```python
from build123d import *

# Parameters (mm, degrees)
F0_W      = 38.1
F0_H      = 38.1
F1_DEPTH  = 38.1
F6_DEPTH  = 38.1
F8_DEPTH  = 38.1
F9_W      = 25.4
F9_H      = 7.62
F10_DEPTH = 38.1


with BuildPart() as f1:
    # F0 (on Front) → F1 (new body)
    with BuildSketch(Plane.XZ):
        with Locations((19.05, 19.05)):
            Rectangle(F0_W, F0_H)
    extrude(amount=F1_DEPTH)

    # F5 (on offset) → F6 (cut)
    with BuildSketch(Plane.YZ.offset(38.1)):
        Polygon((-11.43, 15.875), (-6.35, 38.1), (-31.75, 38.1), (-26.67, 15.875), (-21.59, 28.575), (-16.51, 28.575), align=None)
        Polygon((-31.75, 0), (-38.1, 38.1), (-38.1, 0), align=None)
        Polygon((-25.4, 0), (-12.7, 0), (-19.05, 15.875), align=None)
        Polygon((-6.35, 0), (0, 0), (0, 38.1), align=None)
    extrude(amount=-F6_DEPTH, mode=Mode.SUBTRACT)

    # F7 (on Front) → F8 (cut)
    with BuildSketch(Plane.XZ):
        Polygon((11.43, 22.225), (6.35, 0), (31.75, 0), (26.67, 22.225), (21.59, 9.650744), (16.51, 9.525), align=None)
        Polygon((31.75, 38.1), (38.1, 0), (38.1, 38.1), align=None)
        Polygon((25.4, 38.1), (12.7, 38.1), (19.05, 22.225), align=None)
        Polygon((0, 38.1), (0, 0), (6.35, 38.1), align=None)
    extrude(amount=F8_DEPTH, mode=Mode.SUBTRACT)

    # F9 (on offset) → F10 (cut)
    with BuildSketch(Plane.XY.offset(38.1)):
        with Locations((25.4, -11.43)):
            Rectangle(F9_W, F9_H)
        with Locations((12.7, -26.67)):
            Rectangle(F9_W, F9_H)
    extrude(amount=-F10_DEPTH, mode=Mode.SUBTRACT)


solid = f1.part
```
Build history of the part. All positions in model axes, mm. A direction names the side the tool comes from. Coordinates: 2 decimals unless noted, no trailing zeros. Order: outer loops, then holes, each group sorted by start corner. A loop starts at its lowest first (then second) coordinate and runs counter-clockwise, first axis right, second up. Notation, with made-up numbers: (-25.75, -5.75) -> (21.25, -5.75) arc R24 ccw to (21.25, 6.25) -> close; hole circle Ø3 at (-11, -28). An arc over 180 degrees is marked (long way). Answer in a Markdown table with one row per item. Add a question column.
Q1. Band-saw the part on B-B, the plane z = 4. List the corners of the cut face in (x, y).
Q2. Which spindle directions (+Z, -Z, +X, -X, +Y, -Y) get a long thin tool onto all of the face, cutting with end or side? Do faces 4 (the face through (15.83, -33.39, 30.27)), 5 (the face through (14, -32.4, 15.8)), 6 (the face through (16, -22.86, 18)). Say none if no direction does.
Q3. Wall check: line 1 along Y through (x, z) = (21, 26); line 2 along Y through (x, z) = (32.5, 22); line 3 along Y through (x, z) = (15, 29.5). Give the ranges that are in metal, low to high. Write a range as [from, to].
Q4. Band-saw the part on D-D, the plane z = 20.5. Give the number of separate pieces and of enclosed holes in the cut face, then the cut area to 3 significant figures.
Q5. Band-saw the part on C-C, the plane z = 26.5. List the corners of the cut face in (x, y), then the cut area to 3 significant figures.
Q6. Drop flat-ended pins along their axis: pin 1 (2.5 mm diameter, centred on x = 28, y = -18, fed in from +Z) (3 decimals); pin 2 (8 mm diameter, centred on y = -34, z = 27.5, fed in from +X); pin 3 (3 mm diameter, centred on y = -5, z = 6.5, fed in from +X); pin 4 (6 mm diameter, centred on x = 26, z = 6.5, fed in from +Y) (1 decimal). Give the stop position or say it passes through.
Q7. Mould opens along Y. For faces 1 (the face through (24.166, -5.651, 16.026)), 2 (the face through (19.32, -3.13, 19.32)), 3 (the face through (29.675, -24.166, 22.136)) say: +Y half, -Y half, draft (parallel to the pull), parting line (faces both ways), or undercut.
Answers follow:
| question | item | result |
|---|---|---|
| 1 | outline | (0.67, -32.42) -> (7.26, -32.42) -> (7.26, -30.48) -> (0.67, -30.48) -> close; (0.67, -14.3) -> (7.26, -14.3) -> (7.26, -5.68) -> (0.67, -5.68) -> close; (30.84, -32.42) -> (37.43, -32.42) -> (37.43, -23.8) -> (30.84, -23.8) -> close; (30.84, -7.62) -> (37.43, -7.62) -> (37.43, -5.68) -> (30.84, -5.68) -> close |
| 2 | face 4 | +Z, +Y, -Y |
| 2 | face 5 | -Z, +Y, -Y |
| 2 | face 6 | +Z, -Z, -X |
| 3 | line 1 | [-36.08, -30.48], [-22.62, -15.48], [-7.62, -2.02] |
| 3 | line 2 | [-35.42, -28.07], [-24.22, -15.24], [-7.62, -2.68] |
| 3 | line 3 | [-36.67, -30.48], [-7.62, -1.43] |
| 4 | separate pieces | 9 |
| 4 | enclosed holes | 0 |
| 4 | area | 572 mm^2 |
| 5 | outline | (4.42, -36.17) -> (17.34, -36.17) -> (17.34, -30.48) -> (4.42, -30.48) -> close; (4.42, -22.42) -> (17.34, -22.42) -> (17.34, -15.68) -> (4.42, -15.68) -> close; (4.42, -9) -> (12.7, -9) -> (12.7, -7.62) -> (17.34, -7.62) -> (17.34, -1.93) -> (4.42, -1.93) -> close; (20.76, -36.17) -> (33.68, -36.17) -> (33.68, -29.1) -> (25.4, -29.1) -> (25.4, -30.48) -> (20.76, -30.48) -> close; (20.76, -22.42) -> (33.68, -22.42) -> (33.68, -15.68) -> (20.76, -15.68) -> close; (20.76, -7.62) -> (33.68, -7.62) -> (33.68, -1.93) -> (20.76, -1.93) -> close |
| 5 | area | 491 mm^2 |
| 6 | pin 1 | z = 28.575 |
| 6 | pin 2 | x = 34.18 |
| 6 | pin 3 | x = 37.25 |
| 6 | pin 4 | through |
| 7 | face 1 | draft |
| 7 | face 2 | +Y half |
| 7 | face 3 | undercut |
